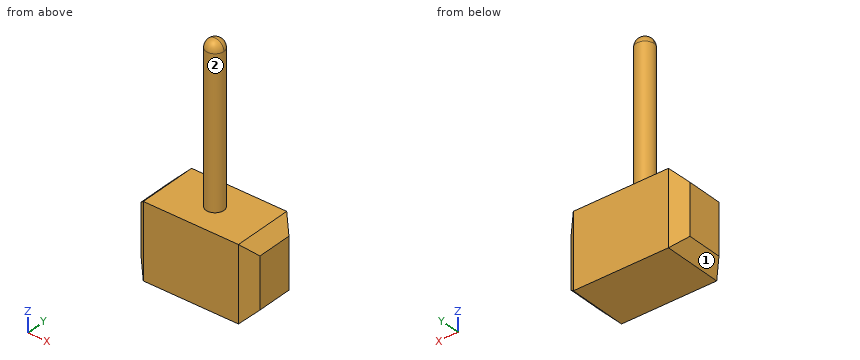
```python
from build123d import *

# Parameters (mm, degrees)
F0_W     = 50.8
F0_H     = 25.4
F1_DEPTH = 31.75
F2_R     = 3.81
F3_DEPTH = 63.5
F6_SIZE  = 5.08
F7_SIZE  = 5.08


with BuildPart() as f1:
    # F0 (on Top) → F1 (new body)
    with BuildSketch(Plane.XY):
        Rectangle(F0_W, F0_H)
    extrude(amount=F1_DEPTH)

    # F2 (on face) → F3 (join)
    with BuildSketch(Plane.XY.offset(31.75)):
        Circle(F2_R)
    extrude(amount=F3_DEPTH)

    # F4 (on face) → F5 (revolve)
    with BuildSketch(Plane.XY.offset(95.25)):
        with BuildLine():
            Line((0, 3.81), (0, -3.81))
            ThreePointArc((0, -3.81), (2.694077, -2.694077), (3.81, 0))
            ThreePointArc((3.81, 0), (2.694077, 2.694077), (0, 3.81))
        make_face()
    revolve(axis=Axis((0, 0, 95.25), (0, -1, 0)))

    # F6
    f6_edges = [f1.edges().sort_by_distance(p)[0] for p in [
        (25.4, 0, 0),
        (25.4, 12.7, 15.875),
        (25.4, 0, 31.75),
        (25.4, -12.7, 15.875),
    ]]
    chamfer(f6_edges, length=F6_SIZE)

    # F7
    f7_edges = [f1.edges().sort_by_distance(p)[0] for p in [
        (-25.4, 0, 31.75),
        (-25.4, 12.7, 15.875),
        (-25.4, -12.7, 15.875),
        (-25.4, 0, 0),
    ]]
    chamfer(f7_edges, length=F7_SIZE)


solid = f1.part
```
The listing builds one solid part. Answer for the finished solid, in the listing's coordinates (mm). Face numbers are marked on the shaded views. A direction names the side the tool comes from. Give positions to 0.01 mm unless a question says otherwise; leave off trailing zeros. Order: outer loops, then holes, each group sorted by start corner. A loop starts at its lowest first (then second) coordinate and runs counter-clockwise, first axis right, second up. Notation, with made-up numbers: (67.5, 81) -> (109.5, 81) arc R9 cw to (109.5, 93) -> close; hole circle Ø5 at (-6.75, 55). An arc over 180 degrees is marked (long way). Answer as CSV lines item,"result". Start each with the question number.
Q1. A cutting plane is placed at B-B (y = -5.75). Determine the outline of the cut face in (x, z).
Q2. Which of the six approach directions +Z, -Z, +X, -X, +Y, -Y give full straight-line access (tool end or side, diameter ignored) to the marked faces 1 and 2?
Q3. Find the intervals of material crossed by L1, parallel to Z at x = -17, y = -9; L2, parallel to X at y = -1.5, z = 36; L3, parallel to Y at x = 1, z = 58, in increasing order.
Q4. Given pin 1 (1 mm diameter, centred on y = -2, z = 29.5, fed in from +X); pin 2 (12 mm diameter, centred on y = 0, z = 37, fed in from +X), each flat-ended and moving along its own axis, determine where each tip first touches the part or whether it passes through.
Q5. A cutting plane is placed at D-D (z = 89). Determine the outline of the cut face in (x, y), then the cut area to 3 significant figures.
Q6. A cutting plane is placed at C-C (x = 8.5). Determine the outline of the cut face in (y, z).
Q7. A cutting plane is placed at A-A (z = 8). Determine the outline of the cut face in (x, y), then the cut area to 3 significant figures.
Results found:
1,outline,"(-25.4, 5.08) -> (-20.32, 0) -> (20.32, 0) -> (25.4, 5.08) -> (25.4, 26.67) -> (20.32, 31.75) -> (-20.32, 31.75) -> (-25.4, 26.67) -> close"
2,face 1,"-Z, -X, +Y, -Y"
2,face 2,"+Z"
3,L1,"0 to 31.75"
3,L2,"-3.5 to 3.5"
3,L3,"-3.68 to 3.68"
4,pin 1,"x = 23.07"
4,pin 2,"x = 21.07"
5,outline,"circle Ø7.62 at (0, 0)"
5,area,"45.6 mm2"
6,outline,"(-12.7, 0) -> (12.7, 0) -> (12.7, 31.75) -> (-12.7, 31.75) -> close"
7,outline,"(-25.4, -7.62) -> (-20.32, -12.7) -> (20.32, -12.7) -> (25.4, -7.62) -> (25.4, 7.62) -> (20.32, 12.7) -> (-20.32, 12.7) -> (-25.4, 7.62) -> close"
7,area,"1,240 mm2"
